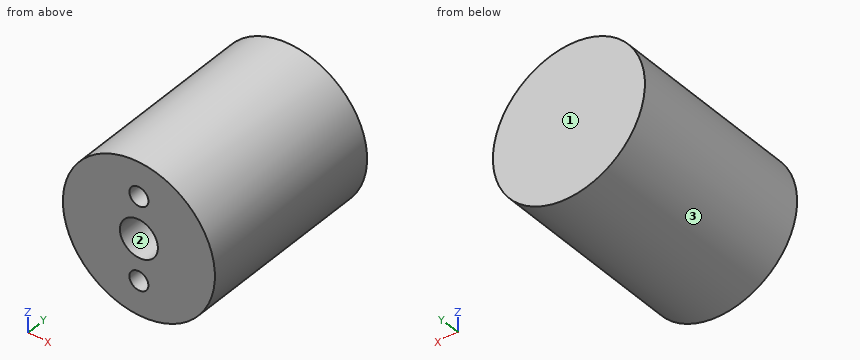
```python
from build123d import *

# Parameters (mm, degrees)
SKETCH1_R           = 40
BOSS_EXTRUDE1_DEPTH = 100
SKETCH2_R           = 10
SKETCH2_R_2         = 5
CUT_EXTRUDE1_DEPTH  = 20


with BuildPart() as part:
    # Sketch1 → Boss-Extrude1 (new body)
    with BuildSketch(Plane(origin=(0, 0, 0), x_dir=(1, 0, 0), z_dir=(0, 1, 0))):
        with Locations(Location((0, 0, 0), (0, 0, 270))):
            Circle(SKETCH1_R)
    extrude(amount=BOSS_EXTRUDE1_DEPTH)

    # Sketch2 → Cut-Extrude1 (cut)
    with BuildSketch(Plane.XZ):
        with Locations(Location((0, 0, 0), (0, 0, 270))):
            Circle(SKETCH2_R)
        with Locations(Location((0, 22, 0), (0, 0, 270))):
            Circle(SKETCH2_R_2)
        with Locations(Location((0, -22, 0), (0, 0, 270))):
            Circle(SKETCH2_R_2)
    extrude(amount=-CUT_EXTRUDE1_DEPTH, mode=Mode.SUBTRACT)


solid = part.part
```
Design review of the part built by this model. Coordinates are the model's own, in mm. Face numbers are marked on the shaded views. Coordinates: 2 decimals unless noted, no trailing zeros. Order: outer loops, then holes, each group sorted by start corner. A loop starts at its lowest first (then second) coordinate and runs counter-clockwise, first axis right, second up. Notation, with made-up numbers: (5.25, 3.5) -> (17.25, 3.5) arc R27 ccw to (17.25, 31.5) -> close; hole circle Ø4 at (73.25, 30). An arc over 180 degrees is marked (long way). One line per item, written item: value. Start each with the question number.
Q1. For probe 1 along X at (y, z) = (12.75, 0); probe 2 along X at (y, z) = (13.25, 22); probe 3 along Y at (x, z) = (2.5, 3), list the stretches that pass through material, from the lowest coordinate up.
Q2. Take a section at A-A, the plane z = 0. State the section outline as (x, y) points, then the cut area to 3 significant figures.
Q3. Take a section at C-C, the plane y = 17. State the section outline as (x, z) points.
Q4. Take a section at B-B, the plane x = 0. State the section outline as (y, z) points, then the cut area to 3 significant figures.
Q5. Take a section at D-D, the plane z = -22. State the section outline as (x, y) points.
Q6. Mouldability with a two-part tool opening along Z and no side actions: class the marked faces 1, 2 and 3 as pulls with the +Z half, pulls with the -Z half, needs draft (parallel to the pull), parting line crosses it, or undercut.
Q7. Insertion check: pin 1 Ø10 at (x, y) = (-21.5, 76) entering from -Z; pin 2 Ø1.5 at (y, z) = (84.5, 19) entering from -X; pin 3 Ø5 at (y, z) = (64.5, -8.5) entering from +X; pin 4 Ø10 at (x, z) = (-2, -5) entering from -Y. Each pin has a flat end and moves straight along its axis. Give the tip position at first contact, or say it passes through.
Values follow:
1. probe 1: x = -40 to -10, 10 to 40
1. probe 2: x = -33.41 to -5, 5 to 33.41
1. probe 3: y = 20 to 100
2. outline: (-40, 0) -> (-10, 0) -> (-10, 20) -> (10, 20) -> (10, 0) -> (40, 0) -> (40, 100) -> (-40, 100) -> close
2. area: 7,600 mm2
3. outline: circle Ø80 at (0, 0); hole circle Ø20 at (0, 0); hole circle Ø10 at (0, -22); hole circle Ø10 at (0, 22)
4. outline: (0, -40) -> (100, -40) -> (100, 40) -> (0, 40) -> (0, 27) -> (20, 27) -> (20, 17) -> (0, 17) -> (0, 10) -> (20, 10) -> (20, -10) -> (0, -10) -> (0, -17) -> (20, -17) -> (20, -27) -> (0, -27) -> close
4. area: 7,200 mm2
5. outline: (-33.41, 0) -> (-5, 0) -> (-5, 20) -> (5, 20) -> (5, 0) -> (33.41, 0) -> (33.41, 100) -> (-33.41, 100) -> close
6. face 1: needs draft
6. face 2: undercut
6. face 3: parting line crosses it
7. pin 1: stops at z = -36.44
7. pin 2: stops at x = -35.59
7. pin 3: stops at x = 39.55
7. pin 4: stops at y = 0
